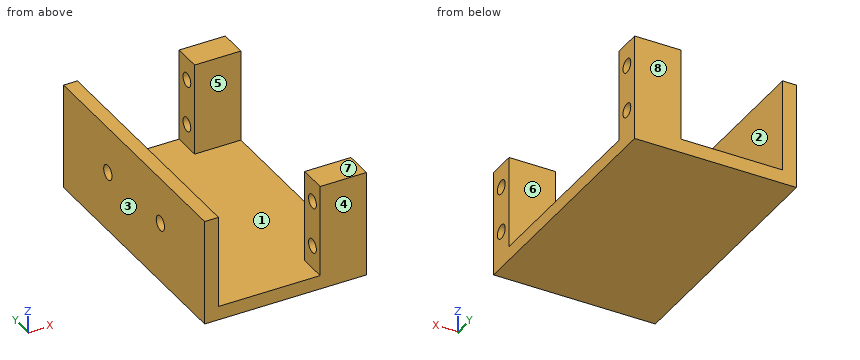
```python
from build123d import *

# Parameters (mm, degrees)
SKETCH_W        = 35
SKETCH_H        = 54.5
PAD_DEPTH       = 3
SKETCH001_W     = 3
SKETCH001_H     = 54.5
PAD001_DEPTH    = 20
SKETCH002_W     = 10
SKETCH002_H     = 6
PAD002_DEPTH    = 20
SKETCH003_R     = 1.5
POCKET_DEPTH    = 11
SKETCH004_R     = 1.6
POCKET001_DEPTH = 5


with BuildPart() as part:
    # Sketch → Pad (new body)
    with BuildSketch(Plane.XY):
        with Locations((17.5, 27.25)):
            Rectangle(SKETCH_W, SKETCH_H)
    extrude(amount=PAD_DEPTH)

    # Sketch001 (on Face6 of Pad) → Pad001 (join)
    with BuildSketch(Plane.XY.offset(3)):
        with Locations((1.5, 27.25)):
            Rectangle(SKETCH001_W, SKETCH001_H)
    extrude(amount=PAD001_DEPTH)

    # Sketch002 (on Face6 of Pad001) → Pad002 (join)
    with BuildSketch(Plane.XY.offset(3)):
        with Locations((30, 3)):
            Rectangle(SKETCH002_W, SKETCH002_H)
        with Locations((30, 51.5)):
            Rectangle(SKETCH002_W, SKETCH002_H)
    extrude(amount=PAD002_DEPTH)

    # Sketch003 (on Face11 of Pad002) → Pocket (cut)
    with BuildSketch(Plane.YZ.offset(35)):
        with Locations((3, 18)):
            Circle(SKETCH003_R)
        with Locations((3, 8)):
            Circle(SKETCH003_R)
        with Locations((51.5, 18)):
            Circle(SKETCH003_R)
        with Locations((51.5, 8)):
            Circle(SKETCH003_R)
    extrude(amount=-POCKET_DEPTH, mode=Mode.SUBTRACT)

    # Sketch004 (on Face12 of Pocket) → Pocket001 (cut)
    with BuildSketch(Plane.YZ.offset(3)):
        with Locations((17.1, 13)):
            Circle(SKETCH004_R)
        with Locations((37.4, 13)):
            Circle(SKETCH004_R)
    extrude(amount=-POCKET001_DEPTH, mode=Mode.SUBTRACT)


solid = part.part
```
Can you work these out from the model? Positions are in its coordinate system, mm. Face numbers are marked on the shaded views. A direction names the side the tool comes from. Coordinates: 2 decimals unless noted, no trailing zeros. Write each loop counter-clockwise with the first axis right and the second up, starting at its lowest first coordinate (ties: lowest second). Pieces come first, ordered by that corner, then holes. Notation, with made-up numbers: (-16.5, -21) - (0.5, -21) arc R26 cw to (0.5, -3) - close; hole circle Ø11 at (37.5, -31.5). An arc over 180 degrees is marked (long way). Return JSON: item names as keys, results as strings.
Q1. On a 3-axis mill with a long thin cutter (end or side, diameter ignored), from which of +Z, -Z, +X, -X, +Y, -Y can I reach the whole of each face in a straight line? I mean the marked faces 1, 2, 3, 4 and 5. Say none if no direction works.
Computed values:
{"face 1": "+Z", "face 2": "+Z, +Y, -Y", "face 3": "+Z, -Z, -X, +Y, -Y", "face 4": "+Z, -Z, +X, -X, -Y", "face 5": "+Z, +X"}
Q2. If we section it at D-D (y = 37.4): Please give me the cut outline in (x, z).
Computed values:
{"outline": "(0, 0) - (35, 0) - (35, 3) - (3, 3) - (3, 11.4) - (0, 11.4) - close; (0, 14.6) - (3, 14.6) - (3, 23) - (0, 23) - close"}
Q3. If we section it at C-C (z = 8): Please give me the cut outline in (x, y), then the cut area to 4 significant figures.
Computed values:
{"outline": "(0, 0) - (3, 0) - (3, 54.5) - (0, 54.5) - close; (25, 0) - (35, 0) - (35, 1.5) - (25, 1.5) - close; (25, 4.5) - (35, 4.5) - (35, 6) - (25, 6) - close; (25, 48.5) - (35, 48.5) - (35, 50) - (25, 50) - close; (25, 53) - (35, 53) - (35, 54.5) - (25, 54.5) - close", "area": "223.5 mm2"}
Q4. If we section it at B-B (y = 3): Please give me the cut outline in (x, z).
Computed values:
{"outline": "(0, 0) - (35, 0) - (35, 6.5) - (25, 6.5) - (25, 3) - (3, 3) - (3, 23) - (0, 23) - close; (25, 9.5) - (35, 9.5) - (35, 16.5) - (25, 16.5) - close; (25, 19.5) - (35, 19.5) - (35, 23) - (25, 23) - close"}
Q5. I'm going to push flat-ended pins straight in: pin 1 Ø1.8 at (y, z) = (4, 11.5) entering from -X; pin 2 Ø12 at (x, y) = (29, 36.5) entering from +Z; pin 3 Ø4 at (y, z) = (37.4, 13) entering from +X. Where does each tip first touch, or does it pass through?
Computed values:
{"pin 1": "stops at x = 0", "pin 2": "stops at z = 3", "pin 3": "stops at x = 3"}
Q6. Please list where these lines run through material, in increasing order: L1, parallel to Z at x = 28.5, y = 3; L2, parallel to Y at x = 29, z = 9.75; L3, parallel to Z at x = 1.7, y = 17.1. Write a range as from..to.
Computed values:
{"L1": "z = 0..6.5, 9.5..16.5, 19.5..23", "L2": "y = 0..6, 48.5..54.5", "L3": "z = 0..11.4, 14.6..23"}
Q7. If we section it at A-A (x = 33): Please give me the cut outline in (y, z).
Computed values:
{"outline": "(0, 0) - (54.5, 0) - (54.5, 23) - (48.5, 23) - (48.5, 3) - (6, 3) - (6, 23) - (0, 23) - close; hole circle Ø3 at (3, 8); hole circle Ø3 at (3, 18); hole circle Ø3 at (51.5, 8); hole circle Ø3 at (51.5, 18)"}
Q8. Thinking about a two-plate mould opening in Y: for the marked faces 6, 7 and 8, which applies, +Y half, -Y half, draft (parallel to the pull), parting line (faces both ways), or undercut?
Computed values:
{"face 6": "undercut", "face 7": "draft", "face 8": "+Y half"}
